CAD build for the part. Positions are in the model's coordinates, mm. A direction names the side the tool comes from. Coordinates: 2 decimals unless noted, no trailing zeros. Order: outer loops, then holes, each group sorted by start corner. A loop starts at its lowest first (then second) coordinate and runs counter-clockwise, first axis right, second up. Notation, with made-up numbers: M -7.75,45.25 L 2.25,45.25 A10 cw 2.25,58.25 Z; hole C 21,47.25 d4. An arc over 180 degrees is marked long. One line per item, written item: value.
from build123d import *
from build123d.topology import SkipClean

# Parameters (mm, degrees)
CROQUIS1_W              = 114
CROQUIS1_H              = 34.2
SALIENTE_EXTRUIR1_DEPTH = 97
VACIADO1_T              = -5
SALIENTE_EXTRUIR2_DEPTH = 97
CORTAR_EXTRUIR1_REACH   = 128.031
CROQUIS3_W              = 13.814275766
CROQUIS3_H              = 40
REDONDEO2_R             = 5
CROQUIS6_W              = 12.3
CROQUIS6_H              = 10.4
CORTAR_EXTRUIR3_DEPTH   = 124.459670354
SALIENTE_EXTRUIR3_DEPTH = 97
CROQUIS8_W              = 13.814275766
CROQUIS8_H              = 40
CORTAR_EXTRUIR4_DEPTH   = 127.030661617
CROQUIS9_W              = 104
CROQUIS9_H              = 87
CORTAR_EXTRUIR5_DEPTH   = 10
CORTAR_EXTRUIR6_START   = -33.316303
CROQUIS11_W             = 1.5
CROQUIS11_H             = 39.999512223
CROQUIS11_H_2           = 40
CORTAR_EXTRUIR6_DEPTH   = 33.316303
CORTAR_EXTRUIR7_START   = -33.316303
CROQUIS13_W             = 15.314275766
CROQUIS13_H             = 4.5
CORTAR_EXTRUIR7_DEPTH   = 33.316303
CROQUIS14_W             = 40
CROQUIS14_H             = 2.980218128
SALIENTE_EXTRUIR4_DEPTH = 15.498885391
CORTAR_EXTRUIR8_DEPTH   = 20.498885391
CROQUIS19_W             = 5
CROQUIS19_H             = 21.536410229
CROQUIS19_H_2           = 2.349460024
SALIENTE_EXTRUIR5_DEPTH = 22
CROQUIS20_W             = 5
CROQUIS20_H             = 36.296521374
SALIENTE_EXTRUIR6_DEPTH = 19.5
CROQUIS21_W             = 87
CROQUIS21_H             = 2.349460024
SALIENTE_EXTRUIR7_DEPTH = 144.815390375
CROQUIS23_W             = 1.39816901
CROQUIS23_H             = 33.700902132
CORTAR_EXTRUIR9_DEPTH   = 95.5
CROQUIS24_W             = 22.493754325
CROQUIS24_H             = 22.211308676
CORTAR_EXTRUIR10_DEPTH  = 1.5
CROQUIS25_W             = 5.544572311
CROQUIS25_H             = 16.748281631
CORTAR_EXTRUIR11_DEPTH  = 1.5
SALIENTE_EXTRUIR8_DEPTH = 46
CROQUIS27_W             = 22
CROQUIS27_H             = 22
CORTAR_EXTRUIR12_DEPTH  = 1
CROQUIS28_W             = 21.106040847
CROQUIS28_H             = 4.330702007
CORTAR_EXTRUIR14_DEPTH  = 1.5


with BuildPart() as part:
    # Croquis1 → Saliente-Extruir1 (new body)
    with BuildSketch(Plane.XY):
        with Locations((0, -8.9)):
            Rectangle(CROQUIS1_W, CROQUIS1_H)
    extrude(amount=-SALIENTE_EXTRUIR1_DEPTH)

    # Vaciado1
    vaciado1_openings = [part.faces().sort_by_distance(p)[0] for p in [
        (0, -26, -48.5),
    ]]
    offset(amount=VACIADO1_T, openings=vaciado1_openings, kind=Kind.INTERSECTION)

    # Croquis2 → Saliente-Extruir2 (add, through all)
    with BuildSketch(Plane(origin=(0, 0, -97), x_dir=(-1, 0, 0), z_dir=(0, 0, -1))):
        Polygon((71.814275766, 8.2), (67.33466189, 8.2), (67.33466189, -3.967393508), (57, -3.967393508), (57, -26), (67.33466189, -26), (71.814275766, -26), align=None)
        Polygon((-57, 8.2), (57, 8.2), (67.33466189, 8.2), (71.814275766, 8.2), (71.814275766, 10.296521374), (-71.814275766, 10.296521374), (-71.814275766, 8.2), (-67.33466189, 8.2), align=None)
        Polygon((-67.33466189, -3.967393508), (-67.33466189, 8.2), (-71.814275766, 8.2), (-71.814275766, -26), (-67.33466189, -26), (-57, -26), (-57, -3.967393508), align=None)
    extrude(amount=-SALIENTE_EXTRUIR2_DEPTH)

    # Croquis3 → Cortar-Extruir1 (cut, up to next)
    with BuildSketch(Plane.XZ.offset(26), mode=Mode.PRIVATE) as cortar_extruir1_sk1:
        with Locations((-61.907137883, -48.5)):
            Rectangle(CROQUIS3_W, CROQUIS3_H)
    cortar_extruir1_tool1 = extrude(cortar_extruir1_sk1.sketch, amount=-CORTAR_EXTRUIR1_REACH, mode=Mode.PRIVATE) & part.part
    # Croquis3 → Cortar-Extruir1 (cut, up to next)
    with BuildSketch(Plane.XZ.offset(26), mode=Mode.PRIVATE) as cortar_extruir1_sk2:
        with Locations((61.907137883, -48.5)):
            Rectangle(CROQUIS3_W, CROQUIS3_H)
    cortar_extruir1_tool2 = extrude(cortar_extruir1_sk2.sketch, amount=-CORTAR_EXTRUIR1_REACH, mode=Mode.PRIVATE) & part.part
    add(cortar_extruir1_tool1.solids().sort_by_distance((-61.907138, -26, -48.5))[0], mode=Mode.SUBTRACT)
    add(cortar_extruir1_tool2.solids().sort_by_distance((61.907138, -26, -48.5))[0], mode=Mode.SUBTRACT)

    # Redondeo2
    # the kernel refuses this fillet: 5 mm, written as the material it takes off along each edge
    with BuildSketch(Plane(origin=(71.814275766, -38.5, -97), x_dir=(0, 0, 1), z_dir=(0, 1, 0)), Plane(origin=(71.814275766, -38.5, 0), x_dir=(-1, 0, 0), z_dir=(0, 1, 0)), Plane(origin=(-71.814275766, 22.796521374, -97), x_dir=(0, 0, 1), z_dir=(0, -1, 0)), Plane(origin=(-71.814275766, 22.796521374, 0), x_dir=(1, 0, 0), z_dir=(0, -1, 0))) as redondeo2_piece_1:
        with BuildLine():
            CenterArc((REDONDEO2_R, -REDONDEO2_R), REDONDEO2_R, 90, 90)
            Line((0, -REDONDEO2_R), (0, 0))
            Line((0, 0), (REDONDEO2_R, 0))
        make_face()
    extrude(amount=61.296521374, mode=Mode.SUBTRACT)

    # Croquis6 → Cortar-Extruir3 (cut, through all)
    with BuildSketch(Plane(origin=(0, 0, -97), x_dir=(-1, 0, 0), z_dir=(0, 0, -1))):
        with Locations((-60.617330945, 2.116303246)):
            Rectangle(CROQUIS6_W, CROQUIS6_H)
        with Locations((60.617330945, 2.116303246)):
            Rectangle(CROQUIS6_W, CROQUIS6_H)
    extrude(amount=-CORTAR_EXTRUIR3_DEPTH, mode=Mode.SUBTRACT)

    # Croquis7 → Saliente-Extruir3 (add, through all)
    with BuildSketch(Plane(origin=(0, 0, -97), x_dir=(-1, 0, 0), z_dir=(0, 0, -1))):
        Polygon((57, 8.2), (57, 7.316303246), (66.667330945, 7.316303246), (66.667330945, -3.083696754), (57, -3.083696754), (57, -3.967393508), (66.814275766, -3.967393508), (67.33466189, -3.967393508), (67.33466189, 8.2), (66.814275766, 8.2), align=None)
        Polygon((-66.667330945, 7.32503221), (-57, 7.32503221), (-57, 8.2), (-66.814275766, 8.2), (-67.33466189, 8.2), (-67.33466189, -3.967393508), (-66.814275766, -3.967393508), (-57, -3.967393508), (-57, -3.083696754), (-66.667330945, -3.083696754), align=None)
    extrude(amount=-SALIENTE_EXTRUIR3_DEPTH)

    # Croquis8 → Cortar-Extruir4 (cut, through all)
    with BuildSketch(Plane(origin=(0, 10.296521374, 0), x_dir=(1, 0, 0), z_dir=(0, 1, 0))):
        with Locations((-61.907137883, 48.5)):
            Rectangle(CROQUIS8_W, CROQUIS8_H)
        with Locations((61.907137883, 48.5)):
            Rectangle(CROQUIS8_W, CROQUIS8_H)
    extrude(amount=-CORTAR_EXTRUIR4_DEPTH, mode=Mode.SUBTRACT)

    # Croquis9 → Cortar-Extruir5 (cut)
    with BuildSketch(Plane.XZ.offset(-3.2)):
        with Locations((0, -48.5)):
            Rectangle(CROQUIS9_W, CROQUIS9_H)
    extrude(amount=-CORTAR_EXTRUIR5_DEPTH, mode=Mode.SUBTRACT)

    # Croquis11 → Cortar-Extruir6 (cut)
    with SkipClean():  # the faces are left unmerged after this step: merging them gives an invalid solid
        with BuildSketch(Plane.XZ.offset(26).offset(CORTAR_EXTRUIR6_START)):
            with Locations((54.25, -48.499756112)):
                Rectangle(CROQUIS11_W, CROQUIS11_H)
            with Locations((-54.25, -48.5)):
                Rectangle(CROQUIS11_W, CROQUIS11_H_2)
        extrude(amount=CORTAR_EXTRUIR6_DEPTH, mode=Mode.SUBTRACT)

    # Croquis13 → Cortar-Extruir7 (cut)
    with BuildSketch(Plane.XZ.offset(26).offset(CORTAR_EXTRUIR7_START)):
        with Locations((-61.157137883, -26.25)):
            Rectangle(CROQUIS13_W, CROQUIS13_H)
        with Locations((-61.157137883, -70.75)):
            Rectangle(CROQUIS13_W, CROQUIS13_H)
        with Locations((61.157137883, -26.25)):
            Rectangle(CROQUIS13_W, CROQUIS13_H)
        with Locations((61.157137883, -70.749512223)):
            Rectangle(CROQUIS13_W, CROQUIS13_H)
    extrude(amount=CORTAR_EXTRUIR7_DEPTH, mode=Mode.SUBTRACT)

    # Croquis14 → Saliente-Extruir4 (add)
    with BuildSketch(Plane.ZY.offset(55)):
        with Locations((-48.5, 8.80641231)):
            Rectangle(CROQUIS14_W, CROQUIS14_H)
    extrude(amount=SALIENTE_EXTRUIR4_DEPTH)

    # Croquis16 → Cortar-Extruir8 (cut)
    with BuildSketch(Plane.ZY.offset(71.814275766)):
        Polygon((-5, 10.296521374), (-98.41592061, 10.296521374), (-98.41592061, -27.13789471), (0, -27.13789471), (0, 10.296521374), align=None)
    extrude(amount=-CORTAR_EXTRUIR8_DEPTH, mode=Mode.SUBTRACT)

    # Croquis19 → Saliente-Extruir5 (add)
    with BuildSketch(Plane.ZY.offset(51.315390375)):
        with Locations((-2.5, -15.231794886)):
            Rectangle(CROQUIS19_W, CROQUIS19_H)
        with Locations((-94.5, -15.231794886)):
            Rectangle(CROQUIS19_W, CROQUIS19_H)
        with Locations((-2.5, 9.121791362)):
            Rectangle(CROQUIS19_W, CROQUIS19_H_2)
        with Locations((-94.5, 9.121791362)):
            Rectangle(CROQUIS19_W, CROQUIS19_H_2)
    extrude(amount=SALIENTE_EXTRUIR5_DEPTH)

    # Croquis20 → Saliente-Extruir6 (add)
    with BuildSketch(Plane.ZY.offset(73.315390375)):
        with Locations((-2.5, -7.851739313)):
            Rectangle(CROQUIS20_W, CROQUIS20_H)
        with Locations((-94.5, -7.851739313)):
            Rectangle(CROQUIS20_W, CROQUIS20_H)
    extrude(amount=SALIENTE_EXTRUIR6_DEPTH)

    # Croquis21 → Saliente-Extruir7 (add)
    with BuildSketch(Plane.ZY.offset(-52)):
        with Locations((-48.5, 9.121791362)):
            Rectangle(CROQUIS21_W, CROQUIS21_H)
    extrude(amount=SALIENTE_EXTRUIR7_DEPTH)

    # Croquis23 → Cortar-Extruir9 (cut)
    with BuildSketch(Plane.XY):
        with Locations((-91.682194084, -7.778032427)):
            Rectangle(CROQUIS23_W, CROQUIS23_H)
    extrude(amount=-CORTAR_EXTRUIR9_DEPTH, mode=Mode.SUBTRACT)

    # Croquis24 → Cortar-Extruir10 (cut)
    with BuildSketch(Plane(origin=(0, 10.296521374, 0), x_dir=(1, 0, 0), z_dir=(0, 1, 0))):
        with Locations((-78.515448222, 48.5)):
            Rectangle(CROQUIS24_W, CROQUIS24_H)
    extrude(amount=-CORTAR_EXTRUIR10_DEPTH, mode=Mode.SUBTRACT)

    # Croquis25 → Cortar-Extruir11 (cut)
    with BuildSketch(Plane(origin=(0, 8.796521374, 0), x_dir=(1, 0, 0), z_dir=(0, 1, 0))):
        with Locations((-86.990039229, 48.639589487)):
            Rectangle(CROQUIS25_W, CROQUIS25_H)
    extrude(amount=-CORTAR_EXTRUIR11_DEPTH, mode=Mode.SUBTRACT)

    # Croquis26 → Saliente-Extruir8 (add)
    with BuildSketch(Plane(origin=(-89.762325384, 0, 0), x_dir=(0, 0, -1), z_dir=(1, 0, 0))):
        Polygon((59.605654338, 10.296521374), (37.394345662, 10.296521374), (37.394345662, 8.796521374), (40.265448671, 8.796521374), (40.265448671, 7.94706135), (57.013730302, 7.94706135), (57.013730302, 8.796521374), (59.605654338, 8.796521374), align=None)
    extrude(amount=SALIENTE_EXTRUIR8_DEPTH)

    # Croquis27 → Cortar-Extruir12 (cut)
    with BuildSketch(Plane(origin=(0, 10.296521374, 0), x_dir=(1, 0, 0), z_dir=(0, 1, 0))):
        with Locations((-71.548762692, 81)):
            Rectangle(CROQUIS27_W, CROQUIS27_H)
    extrude(amount=-CORTAR_EXTRUIR12_DEPTH, mode=Mode.SUBTRACT)

    # Croquis28 → Cortar-Extruir14 (cut)
    with BuildSketch(Plane(origin=(0, 9.296521374, 0), x_dir=(1, 0, 0), z_dir=(0, 1, 0))):
        with Locations((-71.487233446, 89.534648997)):
            Rectangle(CROQUIS28_W, CROQUIS28_H)
    extrude(amount=-CORTAR_EXTRUIR14_DEPTH, mode=Mode.SUBTRACT)


solid = part.part
Q1. Pin check, flat tips, straight feed: pin 1 Ø11 at (x, z) = (-74, -79) entering from +Y; pin 2 Ø12 at (x, z) = (-7.5, -21) entering from -Y; pin 3 Ø1 at (y, z) = (-20.5, -14.5) entering from -X. Stop position of each tip, or through.
Recorded:
pin 1: stops at y = 9.3
pin 2: stops at y = 7.95
pin 3: stops at x = 52
Q2. Slice it at A-A (y = -9.5). List the corners of the cut face in (x, z).
Recorded:
outline: M -92.82,-97 L 66.81,-97 A5 ccw 71.81,-92 L 71.81,-5 A5 ccw 66.81,0 L -90.98,0 L -90.98,-5 L 52,-5 L 52,-92 L -90.98,-92 L -90.98,-95.5 L -92.38,-95.5 L -92.38,-92 L -92.82,-92 Z; M -92.82,-5 L -92.38,-5 L -92.38,0 L -92.82,0 Z; hole M 53.5,-73 L 68.81,-73 L 68.81,-24 L 53.5,-24 Z
Q3. Slice it at C-C (x = 61). List the corners of the cut face in (y, z).
Recorded:
outline: M -26,-97 L -3.08,-97 L -3.08,-73 L -26,-73 Z; M -26,-24 L -3.08,-24 L -3.08,0 L -26,0 Z; M 7.33,-97 L 10.3,-97 L 10.3,-68.5 L 7.33,-68.5 Z; M 7.33,-28.5 L 10.3,-28.5 L 10.3,0 L 7.33,0 Z
Q4. Which spindle directions (+Z, -Z, +X, -X, +Y, -Y) get a long thin tool onto all of the face, cutting with end or side? Do faces 1 (the face through (61, -13, -24)), 2 (the face through (-19, -9, -5)), 3 (the face through (-51.315, 2, -3)). Say none if no direction does.
Recorded:
face 1: -Y
face 2: -X, -Y
face 3: +Z, -Z
Q5. Drill centre lines: line 1 along X through (y, z) = (-17.5, -40.5); line 2 along Z through (x, y) = (-4, -1); line 3 along X through (y, z) = (1.5, -88). Where is each one in solid material? Low to high.
Recorded:
line 1: x = 52 to 53.5, 68.81 to 71.81
line 2: z = -97 to -92, -5 to 0
line 3: x = 52 to 54.47, 66.67 to 71.81
Q6. Slice it at B-B (z = -57). List the corners of the cut face in (x, y).
Recorded:
outline: M -92.82,7.95 L -92.38,7.95 L -92.38,9.07 L -90.98,9.07 L -90.98,7.95 L 52,7.95 L 52,-26 L 53.5,-26 L 53.5,7.32 L 55,7.32 L 55,10.3 L -92.82,10.3 Z; M 68.81,-26 L 71.81,-26 L 71.81,10.3 L 68.81,10.3 Z
Q7. Mould opens along Z. For faces 4 (the face through (-72, 9.297, -79)), 5 (the face through (-12, -8, -97)), 6 (the face through (-62, -4.464, -95)) say: released by +Z, released by -Z, zero draft, split by the parting line, or undercut.
Recorded:
face 4: undercut
face 5: released by -Z
face 6: zero draft
